Source: CAD feature listing. Evaluate the final solid. Frame: model axes, mm. A direction names the side the tool comes from. Give positions to 0.01 mm unless a question says otherwise; leave off trailing zeros. Loops run counter-clockwise (first coordinate to the right, second up) from the corner with the lowest first, then second, coordinate; pieces in that order, holes last. Notation, with made-up numbers: (61, 55.25) -> (83, 55.25) arc R11 ccw to (83, 70.25) -> close; hole circle Ø5 at (-9, 78). An arc over 180 degrees is marked (long way). Put each result on its own line as item: value.
Autodesk Inventor part; units mm, degrees
ref_plane "Work Plane3" through (-11.5, 0, 0) normal (1, 0, 0) x (0, 1, 0)
ref_plane "Work Plane4" through (0, 5, 0) normal (0, 1, 0) x (-1, 0, 0)
ref_plane "Work Plane5" through (0, 0, 6.25) normal (0, 0, 1) x (1, 0, 0)
sketch "Sketch1" plane through (0, 0, 0) normal (0, 1, 0) x (-1, 0, 0)
  line L0 (11.5, -6.25) -> (-11.5, -6.25)
  line L1 (-11.5, -6.25) -> (-11.5, 6.25)
  line L2 (-11.5, 6.25) -> (11.5, 6.25)
  line L3 (11.5, 6.25) -> (11.5, -6.25)
  line L4 (11.5, -6.25) -> (-11.5, 6.25) construction
  line L5 (-11.5, -6.25) -> (11.5, 6.25) construction
  point P0 (0, 0)
  dimension "d0" = 23
  dimension "d1" = 12.5
extrude "Extrusion1" add sketch "Sketch1" along normal mid plane 22
ref_plane "Work Plane3" through (-11.5, 0, 0) normal (1, 0, 0) x (0, 1, 0)
ref_plane "Work Plane2" through (11.5, 0, 0) normal (1, 0, 0) x (0, 1, 0)
ref_plane "Work Plane4" through (0, 5, 0) normal (0, 1, 0) x (-1, 0, 0)
ref_plane "Work Plane5" through (0, 0, 6.25) normal (0, 0, 1) x (1, 0, 0)
sketch "Sketch2" plane through (11.5, -11, -6.25) normal (1, 0, 0) x (0, 0, -1)
  line L0 (0, 0) -> (-12.5, 0)
  line L1 (-12.5, 0) -> (-12.5, 16)
  line L2 (-12.5, 0) -> (-12.5, 22)
  line L3 (-12.5, 16) -> (-15.3, 16)
  line L4 (-15.3, 16) -> (-15.3, 18.5)
  line L5 (-15.3, 18.5) -> (0, 18.5)
  line L6 (0, 18.5) -> (2.8, 18.5)
  line L7 (2.8, 18.5) -> (2.8, 16)
  line L8 (2.8, 16) -> (-12.5, 16)
  point P0 (-6.25, 11)
  dimension "d8" = 16
  dimension "d9" = 2.8
  dimension "d10" = 2.5
  dimension "d11" = 2.8
extrude "Extrusion2" add sketch "Sketch2" along normal blind 4.8
mirror "Mirror1" about plane through (0, 0, 0) normal (1, 0, 0) of "Extrusion2"
ref_plane "Work Plane6" through (0, 11, 0) normal (0, 1, 0) x (-1, 0, 0)
sketch "Sketch3" plane through (0, 11, 0) normal (0, 1, 0) x (-1, 0, 0)
  line L0 (-12.5008, 0) -> (-1.9008, 0)
  arc A0 (3.4585, 2.9134) -> (3.4585, -2.9134) centre (-1.9008, 0) ccw
  circle A1 centre (-1.9008, 0) radius 1
  arc A2 (3.4585, -2.9134) -> (3.4585, 2.9134) centre (4.1992, 0) ccw
  point P0 (0, 0)
  dimension "d15" = 10.6
  dimension "d16" = 12.2
  dimension "d17" = 2
extrude "Extrusion3" add sketch "Sketch3" along normal blind 3.5
sketch "Sketch4" plane through (0, 14.5, 0) normal (0, 1, 0) x (1, 0, 0)
  circle A0 centre (1.9008, 0) radius 1
  circle A1 centre (1.9008, 0) radius 2
  point P0 (0, 0)
  dimension "d20" = 4
extrude "Extrusion4" add sketch "Sketch4" along normal blind 3.2 contours A0 | A1
sketch "Sketch5" plane through (1.9008, 17.7, 0) normal (0, 1, 0) x (1, 0, 0)
  circle A0 centre (0, 0) radius 1
  circle A1 centre (0, 0) radius 1
  point P0 (-1.9008, 0)
extrude "Extrusion5" cut sketch "Sketch5" against normal blind 3.2
sketch "Sketch6" plane through (11.5, 7.5, -6.25) normal (0, 1, 0) x (1, 0, 0)
  circle A0 centre (-9.5992, -6.25) radius 1
  line L0 (-9.5992, -6.25) -> (1.4, -6.25)
  line L1 (4.8, -15.3) -> (4.8, 2.8)
  line L2 (0, -12.5) -> (0, 0)
  line L3 (0, -6.25) -> (4.8, -6.25)
  arc A1 (3.1037, -5.5395) -> (3.1037, -6.9605) centre (2.4, -6.25) ccw
  line L4 (2.4, -5.25) -> (2.4, -5.25)
  line L5 (3.1037, -5.5395) -> (4.8, -5.5395)
  line L6 (3.1037, -6.9605) -> (4.8, -6.9605)
  line L7 (4.8, -6.9605) -> (4.8, -5.5395)
  point P0 (-11.5, -6.25)
  dimension "d25" = 2
extrude "Extrusion6" cut sketch "Sketch6" against normal blind 2.5 contours A1 L5 L1 L3 | L3 L1 L6 A1
mirror "Mirror2" about plane through (0, 0, 0) normal (1, 0, 0) of "Extrusion6"
(1) Section C-C on y = 6.5. Return loops of the section in (x, z).
Calculated:
outline: (-16.3, -9.05) -> (-11.5, -9.05) -> (-11.5, -6.25) -> (11.5, -6.25) -> (11.5, -9.05) -> (16.3, -9.05) -> (16.3, -0.71) -> (14.6, -0.71) arc R1 cw (long way) to (14.6, 0.71) -> (16.3, 0.71) -> (16.3, 9.05) -> (11.5, 9.05) -> (11.5, 6.25) -> (-11.5, 6.25) -> (-11.5, 9.05) -> (-16.3, 9.05) -> (-16.3, 0.71) -> (-14.6, 0.71) arc R1 cw (long way) to (-14.6, -0.71) -> (-16.3, -0.71) -> close
(2) First-contact query: P1, Ø1.5, axis at y = -5.5, z = -5, coming from the -X side; P2, Ø1.2, axis at x = 13.9, z = 0, coming from the +Y side; P3, Ø2, axis at x = -4.5, y = 6, coming from the +Z side; P4, Ø3, axis at x = 9, y = 13, coming from the +Z side. Flat tips, straight axial feed; report the tip coordinate or a pass-through.
Calculated:
P1: stops at x = -11.5
P2: passes through
P3: stops at z = 6.25
P4: stops at z = 2.42
(3) Section B-B on z = 7. Return loops of the section in (x, y).
Calculated:
outline: (-16.3, 5) -> (-11.5, 5) -> (-11.5, 7.5) -> (-16.3, 7.5) -> close; (11.5, 5) -> (16.3, 5) -> (16.3, 7.5) -> (11.5, 7.5) -> close
(4) Section A-A on x = 13.9. Return loops of the section in (y, z), then the cut area to 4 significant figures.
Calculated:
outline: (5, -9.05) -> (7.5, -9.05) -> (7.5, -1) -> (5, -1) -> close; (5, 1) -> (7.5, 1) -> (7.5, 9.05) -> (5, 9.05) -> close
area: 40.25 mm²
(5) Draft query along Z for faces 5 (the flat face through (0, 0, -6.25)), 6 (the flat face through (15, 6, 0.71)), 7 (the flat face through (11.5, -3, 0)). Return one class per face: released by +Z, released by -Z, zero draft, split by the parting line, or undercut.
Calculated:
face 5: released by -Z
face 6: undercut
face 7: zero draft
(6) Line query: probe 1 along X at (y, z) = (14.75, 0); probe 2 along X at (y, z) = (13.5, 0); probe 3 along Z at (x, y) = (13.9, 6.95). Output: solid intervals per line, ascending. Write a range as from..to.
Calculated:
probe 1: x = -0.1..0.9, 2.9..3.9
probe 2: x = -7.21..0.9, 2.9..8
probe 3: z = -9.05..-1, 1..9.05
(7) Reachability of faces 1 (the flat face through (-15, 6, 0.71)), 2 (the flat face through (-11.5, 6, -8)), 3 (the flat face through (-12, 5, 0)), 4 (the flat face through (12, 7.5, 0)) from +Z, -Z, +X, -X, +Y, -Y: full face, straight path, thin tool, end or side. Return the list, or none.
Calculated:
face 1: -X, +Y, -Y
face 2: -Z, +Y, -Y
face 3: +Z, -Z, -X, -Y
face 4: +Z, -Z, +X, +Y
(8) Section D-D on z = 0. Return loops of the section in (x, y).
Calculated:
outline: (-12.9, 5) -> (-11.5, 5) -> (-11.5, -11) -> (11.5, -11) -> (11.5, 5) -> (12.9, 5) -> (12.9, 7.5) -> (11.5, 7.5) -> (11.5, 11) -> (8, 11) -> (8, 14.5) -> (3.9, 14.5) -> (3.9, 17.7) -> (2.9, 17.7) -> (2.9, 11) -> (0.9, 11) -> (0.9, 17.7) -> (-0.1, 17.7) -> (-0.1, 14.5) -> (-7.21, 14.5) -> (-7.21, 11) -> (-11.5, 11) -> (-11.5, 7.5) -> (-12.9, 7.5) -> close
